Read the model definition and answer for the solid it produces. Units are mm, in the model's axes. A direction names the side the tool comes from. Give positions to 0.01 mm unless a question says otherwise; leave off trailing zeros. Loops run counter-clockwise (first coordinate to the right, second up) from the corner with the lowest first, then second, coordinate; pieces in that order, holes last. Notation, with made-up numbers: (-20, -11) - (26, -11) arc R12 cw to (26, 10) - close; hole circle Ø11 at (-14.75, -21.5). An arc over 180 degrees is marked (long way). Write each question's results on one line, items separated by ' | '. Start each with the question number.
Q1. The part is cut by section A-A, the plane x = -5.5. Write down the section's boundary in (y, z).
Q2. The part is cut by section B-B, the plane y = -1. Write down the section's boundary in (x, z).
Q3. Find the intervals of material crossed by line 1 (X direction, y = -15.5, z = -10.5); line 2 (Y direction, x = -1.5, z = -1), in increasing order. Write a range as from..to.
Q4. The part is cut by section C-C, the plane z = -9.75. Write down the section's boundary in (x, y).
Q5. For faces 1 (the flat face through (-10, -11, -6.371)), 2 (the flat face through (5, 1, -12.467)), 3 (the flat face through (-6, -22.098, -9)), determine the directions among +Z, -Z, +X, -X, +Y, -Y from which every point of the face is accessible in a straight line to the end or side of a thin tool.
Q6. The part is cut by section D-D, the plane x = 10. Write down the section's boundary in (y, z), plus the area to 3 significant figures.
Q7. Determine the mould class of faces 4 (the flat face through (6, 2.54, 0)), 5 (the flat face through (-8, -22.86, -9)), 6 (the flat face through (22, -11, -6.371)), 7 (the flat face through (19, -22.098, -9)) for opening direction Y: +Y half, -Y half, draft (parallel to the pull), parting line (faces both ways), or undercut.
Q8. Given pin 1 (12 mm diameter, centred on x = -4, z = 0, fed in from -Y); pin 2 (8 mm diameter, centred on y = -17.5, z = -4, fed in from -X); pin 3 (8 mm diameter, centred on x = 19.5, y = -15, fed in from +Z), each flat-ended and moving along its own axis, determine where each tip first touches the part or whether it passes through.
```python
from build123d import *

# Parameters (mm, degrees)
SKETCH3_W           = 35.56
SKETCH3_H           = 25.4
SKETCH3_R           = 1.778
BOSS_EXTRUDE3_DEPTH = 2.54
SKETCH4_W           = 3.81
SKETCH4_H           = 11.176
BOSS_EXTRUDE4_DEPTH = 22.86
SKETCH5_W           = 11.176
SKETCH5_H           = 0.762
BOSS_EXTRUDE5_DEPTH = 3.302
SKETCH6_W           = 11.176
SKETCH6_H           = 0.762
BOSS_EXTRUDE6_DEPTH = 3.302
SKETCH7_W           = 35.56
SKETCH7_H           = 22.86
CUT_EXTRUDE1_DEPTH  = 5.08


with BuildPart() as part:
    # Sketch3 → Boss-Extrude3 (new body)
    with BuildSketch(Plane(origin=(0, 0, 0), x_dir=(1, 0, 0), z_dir=(0, 1, 0))):
        with Locations((6.262748092, -0.232671756)):
            Rectangle(SKETCH3_W, SKETCH3_H)
        with Locations((-1.674751908, -7.852671756)):
            Circle(SKETCH3_R, mode=Mode.SUBTRACT)
        with Locations((14.200248092, -7.852671756)):
            Circle(SKETCH3_R, mode=Mode.SUBTRACT)
    extrude(amount=BOSS_EXTRUDE3_DEPTH)

    # Sketch4 → Boss-Extrude4 (add)
    with BuildSketch(Plane.XZ):
        with Locations((-9.612251908, -6.879328244)):
            Rectangle(SKETCH4_W, SKETCH4_H)
        with Locations((22.137748092, -6.879328244)):
            Rectangle(SKETCH4_W, SKETCH4_H)
    extrude(amount=BOSS_EXTRUDE4_DEPTH)

    # Sketch5 → Boss-Extrude5 (add)
    with BuildSketch(Plane(origin=(-7.707251908, 0, 0), x_dir=(0, 0, -1), z_dir=(1, 0, 0))):
        with Locations((6.879328244, -22.479)):
            Rectangle(SKETCH5_W, SKETCH5_H)
    extrude(amount=BOSS_EXTRUDE5_DEPTH)

    # Sketch6 → Boss-Extrude6 (add)
    with BuildSketch(Plane.ZY.offset(-20.232748092)):
        with Locations((-6.879328244, -22.479)):
            Rectangle(SKETCH6_W, SKETCH6_H)
    extrude(amount=BOSS_EXTRUDE6_DEPTH)

    # Sketch7 → Cut-Extrude1 (cut)
    with BuildSketch(Plane.XY.offset(-1.291328244)):
        with Locations((6.262748092, -11.43)):
            Rectangle(SKETCH7_W, SKETCH7_H)
    extrude(amount=-CUT_EXTRUDE1_DEPTH, mode=Mode.SUBTRACT)


solid = part.part
```
Check sheet entries:
1) outline: (-22.86, -12.47) - (-22.1, -12.47) - (-22.1, -6.37) - (-22.86, -6.37) - close; (0, -12.47) - (2.54, -12.47) - (2.54, 12.93) - (0, 12.93) - close
2) outline: (-11.52, -12.47) - (-7.71, -12.47) - (-7.71, -6.37) - (-11.52, -6.37) - close; (20.23, -12.47) - (24.04, -12.47) - (24.04, -6.37) - (20.23, -6.37) - close
3) line 1: x = -11.52..-7.71, 20.23..24.04 | line 2: y = 0..2.54
4) outline: (-11.52, -22.86) - (-4.41, -22.86) - (-4.41, -22.1) - (-7.71, -22.1) - (-7.71, 0) - (20.23, 0) - (20.23, -22.1) - (16.93, -22.1) - (16.93, -22.86) - (24.04, -22.86) - (24.04, 2.54) - (-11.52, 2.54) - close
5) face 1: +Z, +X, -X, -Y | face 2: -Z, +X, -X, +Y, -Y | face 3: +Z, -Z
6) outline: (0, -12.47) - (2.54, -12.47) - (2.54, 12.93) - (0, 12.93) - close | area: 64.5 mm^2
7) face 4: +Y half | face 5: -Y half | face 6: draft | face 7: undercut
8) pin 1: stops at y = 0 | pin 2: stops at x = -11.52 | pin 3: stops at z = -6.37
